Here's how the part is built. I have some questions about the finished solid (model axes, mm). A direction names the side the tool comes from. Round coordinates to 2 decimals unless told otherwise and drop trailing zeros. Write each loop counter-clockwise with the first axis right and the second up, starting at its lowest first coordinate (ties: lowest second). Pieces come first, ordered by that corner, then holes. Notation, with made-up numbers: (-9.5, 37.5) - (32.5, 37.5) arc R22 ccw to (32.5, 53.5) - close; hole circle Ø3 at (60.25, 19). An arc over 180 degrees is marked (long way). One line per item, written item: value. Start each with the question number.
Item 1: Imagine slicing it at B-B, the plane y = 325. Please give me the cut outline in (x, z), then the cut area to 3 significant figures.
Item 2: For P1, Ø8, axis at x = 74, y = 8, coming from the -Z side; P2, Ø8, axis at y = 346.41, z = -200, coming from the +X side; P3, Ø8.5, axis at y = -95.26, z = -55, coming from the -X side; P4, Ø1.5, axis at x = 29, z = 26, coming from the +Y side, each with a flat end and sliding along its axis, tell me the tip position at first contact or that it passes through.
Item 3: If I drill on line 1 (Y direction, x = 11.25, z = 88.5); line 2 (Y direction, x = 5.25, z = 118.5); line 3 (Z direction, x = 9, y = 72.5), over which ranges is the centre line in solid material (lowest first)?
Item 4: Thinking about a two-plate mould opening in Y: for faces 4 (the face through (-23, -18, -58)), 5 (the face through (5.98, -53, 4)), 6 (the face through (7.6, 287.24, 313.24)), which applies, released by +Y, released by -Y, zero draft, split by the parting line, or undercut?
Item 5: Imagine slicing it at A-A, the plane z = -224. Please give me the cut outline in (x, y), then the cut area to 3 significant figures.
Item 6: For faces 1 (the face through (85, 2, -56)), 2 (the face through (15, 100, -100)), 3 (the face through (-11.339, -51.721, -67.453)), which set-ups out of +Z, -Z, +X, -X, +Y, -Y let a thin tool reach every point of the face, with its end or its side?
```python
from build123d import *

# Parameters (mm, degrees)
SKETCH1_W                    = 15
SKETCH1_H                    = 425
SKETCH2_R                    = 140
BOSS_EXTRUDE1_DEPTH          = 20
SKETCH3_R                    = 130
BOSS_EXTRUDE2_DEPTH          = 50
SKETCH4_R                    = 85
BOSS_EXTRUDE3_DEPTH          = 23
F_1_4_CLEARANCE_HOLE1_D      = 6.647
F_1_4_CLEARANCE_HOLE1_DEPTH  = 85
HOLE1_D                      = 13
HOLE1_DEPTH                  = 85
HOLE1_TIP                    = 3.905594024
HOLE2_D                      = 10.5
HOLE2_DEPTH                  = 85
HOLE2_TIP                    = 3.15451825
F_5_16_CLEARANCE_HOLE1_D     = 8.376
F_5_16_CLEARANCE_HOLE1_DEPTH = 85
HOLE3_D                      = 95
HOLE3_DEPTH                  = 38
HOLE4_D                      = 106
HOLE4_CBORE_D                = 120
HOLE4_CBORE_DEPTH            = 28.979995345


with BuildPart() as part:
    # Sketch1 → Revolve1 (revolve)
    with BuildSketch(Plane.XY, mode=Mode.PRIVATE) as revolve1_sk:
        with Locations((7.5, 212.5)):
            Rectangle(SKETCH1_W, SKETCH1_H)
    revolve(revolve1_sk.sketch.rotate(Axis((0, 0, 0), (1, 0, 0)), 270), axis=Axis((0, 0, 0), (1, 0, 0)))

    # Sketch2 → Boss-Extrude1 (add)
    with BuildSketch(Plane(origin=(15, 0, 0), x_dir=(0, 0, -1), z_dir=(1, 0, 0))):
        Circle(SKETCH2_R)
    extrude(amount=BOSS_EXTRUDE1_DEPTH)

    # Sketch3 → Boss-Extrude2 (add)
    with BuildSketch(Plane(origin=(35, 0, 0), x_dir=(0, 0, -1), z_dir=(1, 0, 0))):
        Circle(SKETCH3_R)
    extrude(amount=BOSS_EXTRUDE2_DEPTH)

    # Sketch4 → Boss-Extrude3 (add)
    with BuildSketch(Plane.ZY):
        Circle(SKETCH4_R)
    extrude(amount=BOSS_EXTRUDE3_DEPTH)

    # Sketch5 → Cut-Revolve1 (revolve, cut)
    with BuildSketch(Plane(origin=(0, 0, 0), x_dir=(-1, 0, 0), z_dir=(0, 0, -1)), mode=Mode.PRIVATE) as cut_revolve1_sk:
        Polygon((-85, 113.3235), (-85, 110), (-67, 110), (-68.996960267, 113.3235), (-73, 113.3235), align=None)
    revolve(cut_revolve1_sk.sketch.rotate(Axis((85, 110, 0), (-1, 0, 0)), 90), axis=Axis((85, 110, 0), (-1, 0, 0)), mode=Mode.SUBTRACT)

    # Sketch6 → Cut-Revolve2 (revolve, cut)
    with BuildSketch(Plane(origin=(0, 0, -55), x_dir=(-1, 0, 0), z_dir=(0, 0, -1)), mode=Mode.PRIVATE) as cut_revolve2_sk:
        Polygon((-85, 98.586294416), (-85, 95.262794416), (-67, 95.262794416), (-68.996960267, 98.586294416), (-73, 98.586294416), align=None)
    revolve(cut_revolve2_sk.sketch.rotate(Axis((85, 95.262794416, -55), (-1, 0, 0)), 90), axis=Axis((85, 95.262794416, -55), (-1, 0, 0)), mode=Mode.SUBTRACT)

    # Sketch7 → Cut-Revolve3 (revolve, cut)
    with BuildSketch(Plane(origin=(0, 0, -95.262794416), x_dir=(-1, 0, 0), z_dir=(0, 0, -1)), mode=Mode.PRIVATE) as cut_revolve3_sk:
        Polygon((-85, 58.3235), (-85, 55), (-67, 55), (-68.996960267, 58.3235), (-73, 58.3235), align=None)
    revolve(cut_revolve3_sk.sketch.rotate(Axis((85, 55, -95.262794416), (-1, 0, 0)), 90), axis=Axis((85, 55, -95.262794416), (-1, 0, 0)), mode=Mode.SUBTRACT)

    # Sketch8 → Cut-Revolve4 (revolve, cut)
    with BuildSketch(Plane(origin=(0, 0, -110), x_dir=(-1, 0, 0), z_dir=(0, 0, -1)), mode=Mode.PRIVATE) as cut_revolve4_sk:
        Polygon((-85, 3.3235), (-85, 0), (-67, 0), (-68.996960267, 3.3235), (-73, 3.3235), align=None)
    revolve(cut_revolve4_sk.sketch.rotate(Axis((85, 0, -110), (-1, 0, 0)), 90), axis=Axis((85, 0, -110), (-1, 0, 0)), mode=Mode.SUBTRACT)

    # Sketch9 → Cut-Revolve5 (revolve, cut)
    with BuildSketch(Plane(origin=(0, 0, -95.262794416), x_dir=(-1, 0, 0), z_dir=(0, 0, -1)), mode=Mode.PRIVATE) as cut_revolve5_sk:
        Polygon((-85, -51.6765), (-85, -55), (-67, -55), (-68.996960267, -51.6765), (-73, -51.6765), align=None)
    revolve(cut_revolve5_sk.sketch.rotate(Axis((85, -55, -95.262794416), (-1, 0, 0)), 90), axis=Axis((85, -55, -95.262794416), (-1, 0, 0)), mode=Mode.SUBTRACT)

    # Sketch10 → Cut-Revolve6 (revolve, cut)
    with BuildSketch(Plane(origin=(0, 0, -55), x_dir=(-1, 0, 0), z_dir=(0, 0, -1)), mode=Mode.PRIVATE) as cut_revolve6_sk:
        Polygon((-85, -91.939294416), (-85, -95.262794416), (-67, -95.262794416), (-68.996960267, -91.939294416), (-73, -91.939294416), align=None)
    revolve(cut_revolve6_sk.sketch.rotate(Axis((85, -95.262794416, -55), (-1, 0, 0)), 90), axis=Axis((85, -95.262794416, -55), (-1, 0, 0)), mode=Mode.SUBTRACT)

    # Sketch11 → Cut-Revolve7 (revolve, cut)
    with BuildSketch(Plane(origin=(0, 0, 0), x_dir=(-1, 0, 0), z_dir=(0, 0, -1)), mode=Mode.PRIVATE) as cut_revolve7_sk:
        Polygon((-85, -106.6765), (-85, -110), (-67, -110), (-68.996960267, -106.6765), (-73, -106.6765), align=None)
    revolve(cut_revolve7_sk.sketch.rotate(Axis((85, -110, 0), (-1, 0, 0)), 90), axis=Axis((85, -110, 0), (-1, 0, 0)), mode=Mode.SUBTRACT)

    # Sketch12 → Cut-Revolve8 (revolve, cut)
    with BuildSketch(Plane(origin=(0, 0, 55), x_dir=(-1, 0, 0), z_dir=(0, 0, -1)), mode=Mode.PRIVATE) as cut_revolve8_sk:
        Polygon((-85, -91.939294416), (-85, -95.262794416), (-67, -95.262794416), (-68.996960267, -91.939294416), (-73, -91.939294416), align=None)
    revolve(cut_revolve8_sk.sketch.rotate(Axis((85, -95.262794416, 55), (-1, 0, 0)), 90), axis=Axis((85, -95.262794416, 55), (-1, 0, 0)), mode=Mode.SUBTRACT)

    # Sketch13 → Cut-Revolve9 (revolve, cut)
    with BuildSketch(Plane(origin=(0, 0, 95.262794416), x_dir=(-1, 0, 0), z_dir=(0, 0, -1)), mode=Mode.PRIVATE) as cut_revolve9_sk:
        Polygon((-85, -51.6765), (-85, -55), (-67, -55), (-68.996960267, -51.6765), (-73, -51.6765), align=None)
    revolve(cut_revolve9_sk.sketch.rotate(Axis((85, -55, 95.262794416), (-1, 0, 0)), 90), axis=Axis((85, -55, 95.262794416), (-1, 0, 0)), mode=Mode.SUBTRACT)

    # Sketch14 → Cut-Revolve10 (revolve, cut)
    with BuildSketch(Plane(origin=(0, 0, 110), x_dir=(-1, 0, 0), z_dir=(0, 0, -1)), mode=Mode.PRIVATE) as cut_revolve10_sk:
        Polygon((-85, 3.3235), (-85, 0), (-67, 0), (-68.996960267, 3.3235), (-73, 3.3235), align=None)
    revolve(cut_revolve10_sk.sketch.rotate(Axis((85, 0, 110), (-1, 0, 0)), 90), axis=Axis((85, 0, 110), (-1, 0, 0)), mode=Mode.SUBTRACT)

    # Sketch15 → Cut-Revolve11 (revolve, cut)
    with BuildSketch(Plane(origin=(0, 0, 95.262794416), x_dir=(-1, 0, 0), z_dir=(0, 0, -1)), mode=Mode.PRIVATE) as cut_revolve11_sk:
        Polygon((-85, 58.3235), (-85, 55), (-67, 55), (-68.996960267, 58.3235), (-73, 58.3235), align=None)
    revolve(cut_revolve11_sk.sketch.rotate(Axis((85, 55, 95.262794416), (-1, 0, 0)), 90), axis=Axis((85, 55, 95.262794416), (-1, 0, 0)), mode=Mode.SUBTRACT)

    # Sketch16 → Cut-Revolve12 (revolve, cut)
    with BuildSketch(Plane(origin=(0, 0, 55), x_dir=(-1, 0, 0), z_dir=(0, 0, -1)), mode=Mode.PRIVATE) as cut_revolve12_sk:
        Polygon((-85, 98.586294416), (-85, 95.262794416), (-67, 95.262794416), (-68.996960267, 98.586294416), (-73, 98.586294416), align=None)
    revolve(cut_revolve12_sk.sketch.rotate(Axis((85, 95.262794416, 55), (-1, 0, 0)), 90), axis=Axis((85, 95.262794416, 55), (-1, 0, 0)), mode=Mode.SUBTRACT)

    # 1_4 Clearance Hole1
    with Locations(Plane.ZY):
        with Locations((88.5, -218.5), (88.5, -149.231363996), (44.25, -218.5), (0, -218.5), (-44.25, -218.5), (150.255407557, -86.75), (-88.5, -218.5), (-88.5, -149.231363996), (-173.5, 0), (-150.255407557, -86.75), (-157.244401051, 73.324268412), (-118.5, 126.7280553), (-118.5, 185.11402765), (-118.5, 243.5), (-59.25, 243.5), (0, 243.5), (59.25, 243.5), (118.5, 243.5), (118.5, 185.11402765), (118.5, 126.7280553), (157.244401051, 73.324268412), (173.5, 0)):
            Hole(F_1_4_CLEARANCE_HOLE1_D / 2, depth=F_1_4_CLEARANCE_HOLE1_DEPTH)

    # Hole1
    with Locations(Plane.ZY):
        with Locations((400, 0), (346.410161514, -200), (200, -346.410161514), (0, -400), (-200, -346.410161514), (-346.410161514, -200), (-400, 0), (-346.410161514, 200), (-200, 346.410161514), (0, 400), (200, 346.410161514), (346.410161514, 200)):
            Hole(HOLE1_D / 2, depth=HOLE1_DEPTH)
            with Locations((0, 0, -(HOLE1_DEPTH + HOLE1_TIP / 2))):  # 118° drill point
                Cone(0, HOLE1_D / 2, HOLE1_TIP, mode=Mode.SUBTRACT)

    # Hole2
    with Locations(Plane.ZY):
        with Locations((0, -345), (-172.5, -298.778764306), (-298.778764306, -172.5), (-345, 0), (-298.778764306, 172.5), (-172.5, 298.778764306), (0, 345), (172.5, 298.778764306), (298.778764306, 172.5), (345, 0), (298.778764306, -172.5), (172.5, -298.778764306)):
            Hole(HOLE2_D / 2, depth=HOLE2_DEPTH)
            with Locations((0, 0, -(HOLE2_DEPTH + HOLE2_TIP / 2))):  # 118° drill point
                Cone(0, HOLE2_D / 2, HOLE2_TIP, mode=Mode.SUBTRACT)

    # 5_16 Clearance Hole1
    with Locations(Plane.ZY):
        with Locations((266.932809898, -185.615530061), (185.615530061, -266.932809898), (104.298250225, -185.615530061), (185.615530061, -104.298250225), (185.615530061, -185.615530061), (242.974289503, -181.587786851)):
            Hole(F_5_16_CLEARANCE_HOLE1_D / 2, depth=F_5_16_CLEARANCE_HOLE1_DEPTH)

    # Hole3
    with Locations(Plane(origin=(15, 0, 0), x_dir=(0, 0, -1), z_dir=(1, 0, 0))):
        with Locations((-185.615530061, -185.615530061)):
            Hole(HOLE3_D / 2, depth=HOLE3_DEPTH)

    # Hole4 (through all)
    with Locations(Plane.ZY.offset(23)):
        with Locations((0, 0)):
            CounterBoreHole(HOLE4_D / 2, HOLE4_CBORE_D / 2, HOLE4_CBORE_DEPTH)


solid = part.part
```
Values follow:
1. outline: (0, -273.86) - (15, -273.86) - (15, 273.86) - (0, 273.86) - close
1. area: 8,220 mm^2
2. P1: stops at z = -129.94
2. P2: passes through
2. P3: stops at x = 0
2. P4: stops at y = 137.7
3. line 1: y = -415.68 to -221.82, -215.18 to -152.55, -145.91 to 415.68
3. line 2: y = -408.15 to 123.4, 130.05 to 181.79, 188.44 to 240.18, 246.82 to 408.15
3. line 3: z = -418.77 to -160.46, -154.02 to 154.02, 160.46 to 418.77
4. face 4: zero draft
4. face 5: undercut
4. face 6: split by the parting line
5. outline: (0, -361.18) - (15, -361.18) - (15, 361.18) - (0, 361.18) - close
5. area: 10,800 mm^2
6. face 1: +Z, -Z, +X, +Y, -Y
6. face 2: +X
6. face 3: -X
